Autodesk Inventor part; units mm, degrees
ref_plane "YZ Plane" through (0, 0, 0) normal (1, 0, 0) x (0, 1, 0)
ref_plane "XZ Plane" through (0, 0, 0) normal (0, 1, 0) x (-1, 0, 0)
ref_plane "XY Plane" through (0, 0, 0) normal (0, 0, 1) x (1, 0, 0)
sketch "Sketch1" plane through (0, 0, 0) normal (0, 1, 0) x (-1, 0, 0)
  line L0 (0, 0) -> (0, 20)
  line L1 (0, 20) -> (60, 20)
  line L2 (60, 20) -> (66.9645, 38.7482)
  line L3 (66.9645, 38.7482) -> (71.6515, 37.0071)
  line L4 (71.6515, 37.0071) -> (63.1538, 13.4957)
  line L5 (63.1538, 13.4957) -> (8.1538, 13.4957)
  line L6 (8.1538, 13.4957) -> (8.1538, 0)
  line L7 (8.1538, 0) -> (0, 0)
  dimension "d0" = 20
  dimension "d1" = 60
  dimension "d2" = 20
  dimension "d3" = 5
  dimension "d4" = 25
  dimension "d5" = 55
extrude "Extrusion1" add sketch "Sketch1" along normal blind 40
sketch "Sketch2" plane through (0, 40, 0) normal (0, 1, 0) x (1, 0, 0)
  point P0 (0, 0)
properties part number "montageArm"
The model under review builds one solid part; all positions refer to its coordinate system, in mm. A direction names the side the tool comes from. Give positions to 0.01 mm unless a question says otherwise; leave off trailing zeros. Write each loop counter-clockwise with the first axis right and the second up, starting at its lowest first coordinate (ties: lowest second). Pieces come first, ordered by that corner, then holes.
(1) Tool access review of faces 1 (the flat face through (-8.154, 20, 7)), 2 (the flat face through (-30, 20, 20)), 3 (the flat face through (-4, 20, 0)): name each direction out of +Z, -Z, +X, -X, +Y, -Y from which nothing blocks a thin tool from reaching the whole face with its end or side.
(2) To check wall thickness, follow L1, parallel to Z at x = -38, y = 11; L2, parallel to X at y = 30, z = 8; L3, parallel to Z at x = -7, y = 27.5. State the ranges of each line that lie inside material, in increasing order.
(3) Consider section B-B, the plane x = -47. Give the boundary of the cut face in (y, z).
(4) For P1, Ø6, axis at x = -21, y = 5.5, coming from the -Z side; P2, Ø11, axis at y = 12, z = 5, coming from the -X side; P3, Ø3, axis at y = 29.5, z = 30.5, coming from the +X side, all flat-tipped, find the tip position at first contact; note any pin that passes through.
(5) Consider section C-C, the plane z = 30.5. Give the boundary of the cut face in (x, y).
(6) Consider section A-A, the plane y = 16.5. Give the boundary of the cut face in (x, z), and give its area (3 significant figures).
Returned:
1. face 1: -Z, -X, +Y, -Y
1. face 2: +Z, +X, +Y, -Y
1. face 3: -Z, +X, -X, +Y, -Y
2. L1: z = 13.5 to 20
2. L2: x = -8.15 to 0
2. L3: z = 0 to 20
3. outline: (0, 13.5) - (40, 13.5) - (40, 20) - (0, 20) - close
4. P1: stops at z = 13.5
4. P2: stops at x = -8.15
4. P3: stops at x = -63.34
5. outline: (-69.3, 0) - (-63.9, 0) - (-63.9, 40) - (-69.3, 40) - close
6. outline: (-71.65, 37.01) - (-63.15, 13.5) - (-8.15, 13.5) - (-8.15, 0) - (0, 0) - (0, 20) - (-60, 20) - (-66.96, 38.75) - close
6. area: 625 mm2
